from build123d import *

# Parameters (mm, degrees)
SKETCH2_OUTSIDE_W  = 80.304
SKETCH2_OUTSIDE_H  = 80.304
SKETCH2_OUTSIDE_R  = 1.59
CUT_EXTRUDE1_DEPTH = 24.62


with BuildPart() as part:
    # Sketch1 → Revolve1 (revolve)
    with BuildSketch(Plane.XY, mode=Mode.PRIVATE) as revolve1_sk:
        Polygon((0, 0), (0, 8.725), (10.67, 8.725), (10.67, 30), (13.06, 30), (13.06, 9.4), (34.29, 9.4), (34.29, 0), align=None)
    revolve(revolve1_sk.sketch.rotate(Axis((0, 0, 0), (1, 0, 0)), 90), axis=Axis((0, 0, 0), (1, 0, 0)))  # turned: the seam where the file's is

    # Sketch2 outside → Cut-Extrude1 (cut, through all)
    with BuildSketch(Plane.ZY.offset(-10.67)):
        Rectangle(SKETCH2_OUTSIDE_W, SKETCH2_OUTSIDE_H)
        with BuildLine():
            Line((-11.29, 14.29), (11.29, 14.29))
            ThreePointArc((11.29, 14.29), (13.411320344, 13.411320344), (14.29, 11.29))
            Line((14.29, 11.29), (14.29, -11.29))
            ThreePointArc((14.29, -11.29), (13.411320344, -13.411320344), (11.29, -14.29))
            Line((11.29, -14.29), (-11.29, -14.29))
            ThreePointArc((-11.29, -14.29), (-13.411320344, -13.411320344), (-14.29, -11.29))
            Line((-14.29, -11.29), (-14.29, 11.29))
            ThreePointArc((-14.29, 11.29), (-13.411320344, 13.411320344), (-11.29, 14.29))
        make_face(mode=Mode.SUBTRACT)
        with Locations((10.72, 10.72)):
            Circle(SKETCH2_OUTSIDE_R)
        with Locations((-10.72, 10.72)):
            Circle(SKETCH2_OUTSIDE_R)
        with Locations((-10.72, -10.72)):
            Circle(SKETCH2_OUTSIDE_R)
        with Locations((10.72, -10.72)):
            Circle(SKETCH2_OUTSIDE_R)
    extrude(amount=-CUT_EXTRUDE1_DEPTH, mode=Mode.SUBTRACT)


solid = part.part
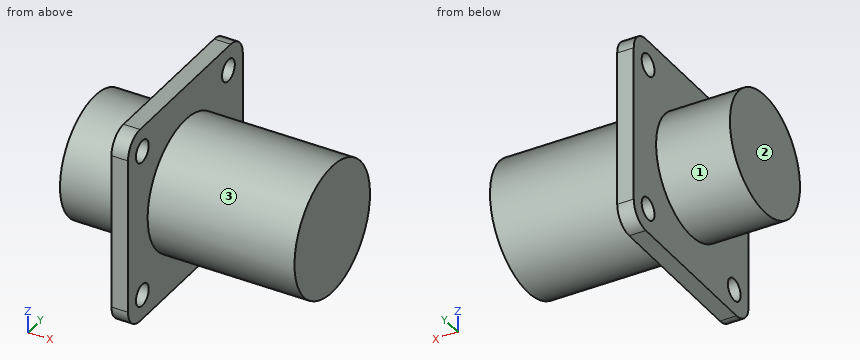
Check sheet for the modelled part. Datum: model origin and axes. Units: mm. Face numbers are marked on the shaded views. A direction names the side the tool comes from. Round coordinates to 2 decimals unless told otherwise and drop trailing zeros. Order: outer loops, then holes, each group sorted by start corner. A loop starts at its lowest first (then second) coordinate and runs counter-clockwise, first axis right, second up.
Q1. Cross-section at D-D, the plane x = 20. Enter the section's corners in (y, z), plus the area to 3 significant figures.
Filled sheet:
outline: circle Ø18.8 at (0, 0)
area: 278 mm2
Q2. Scan lines: L1, parallel to Y at x = 12.1, z = -10.72; L2, parallel to X at y = 6.5, z = -11.75; L3, parallel to Y at x = 12, z = 11.25. Record each from-to range of solid material in increasing order.
Filled sheet:
L1: y = -14.29 to -12.31, -9.13 to 9.13, 12.31 to 14.29
L2: x = 10.67 to 13.06
L3: y = -14.29 to -12.22, -9.22 to 9.22, 12.22 to 14.29
Q3. Set-up check for the marked faces 1, 2 and 3: record each of +Z, -Z, +X, -X, +Y, -Y from which the full face is reachable in a straight line by a thin tool's end or side.
Filled sheet:
face 1: -X
face 2: +Z, -Z, -X, +Y, -Y
face 3: +X
Q4. Cross-section at C-C, the plane y = 0. Enter the section's corners in (x, z) (3 decimals).
Filled sheet:
outline: (0, -8.725) - (10.67, -8.725) - (10.67, -14.29) - (13.06, -14.29) - (13.06, -9.4) - (34.29, -9.4) - (34.29, 9.4) - (13.06, 9.4) - (13.06, 14.29) - (10.67, 14.29) - (10.67, 8.725) - (0, 8.725) - close
Q5. Cross-section at A-A, the plane y = 10.72. Enter the section's corners in (x, z), plus the area to 3 significant figures.
Filled sheet:
outline: (10.67, -14.29) - (13.06, -14.29) - (13.06, -12.31) - (10.67, -12.31) - close; (10.67, -9.13) - (13.06, -9.13) - (13.06, 9.13) - (10.67, 9.13) - close; (10.67, 12.31) - (13.06, 12.31) - (13.06, 14.29) - (10.67, 14.29) - close
area: 53.1 mm2
Q6. Depth check by flat-ended pin: P1, Ø3.5, axis at y = 10.72, z = -10.72, coming from the -X side; P2, Ø10, axis at x = 25.5, y = -10.5, coming from the +Z side; P3, Ø4, axis at x = 28.5, y = 6, coming from the +Z side; P4, Ø1.9, axis at y = -10.72, z = 10.72, coming from the -X side. Enter the tip coordinate at first touch or a pass-through.
Filled sheet:
P1: stops at x = 10.67
P2: stops at z = 7.62
P3: stops at z = 8.51
P4: passes through
